Model file for the job. Use its own axes, mm. Coordinates: 2 decimals unless noted, no trailing zeros. Order: outer loops, then holes, each group sorted by start corner. A loop starts at its lowest first (then second) coordinate and runs counter-clockwise, first axis right, second up. Notation, with made-up numbers: (17.25, -2) -> (32.25, -2) arc R26 cw to (32.25, 24) -> close; hole circle Ø2 at (49, 4). An arc over 180 degrees is marked (long way). Use CSV: the item, a comma, the result in double quotes. Start each with the question number.
(1) Probe L1, parallel to Y at x = 1.25, z = 7; L2, parallel to Y at x = -2.25, z = 15.25; L3, parallel to Z at x = 3.75, y = 2.5. List the from-to ranges inside material, lowest first.
(2) Cut at C-C on z = 16. Write the cut outline in (x, y).
(3) Pin check, flat tips, straight feed: pin 1 Ø3 at (x, y) = (0.5, -7.5) entering from +Z; pin 2 Ø5 at (x, z) = (-3.5, 10.5) entering from +Y; pin 3 Ø3 at (y, z) = (0.61, 6.83) entering from -X; pin 4 Ø1 at (x, y) = (-1, 8.5) entering from -Z. Stop position of each tip, or through.
(4) Cut at B-B on z = 7.5. Write the cut outline in (x, y).
(5) Pull direction Z, two halves, no side cores. Call faces 1 (the flat face through (4.178, 3.3, 7)), 2 (the cylindrical face through (-1.74, 7.59, -0.32)): pulls with the +Z half, pulls with the -Z half, needs draft (parallel to the pull), parting line crosses it, or undercut.
(6) Cut at D-D on y = -5.5. Write the cut outline in (x, z), plus the area to 3 significant figures.
(7) Cut at A-A on y = -8. Write the cut outline in (x, z).
```python
from build123d import *

# Parameters (mm, degrees)
SKETCH1_R           = 2.5
BOSS_EXTRUDE1_DEPTH = 12
BOSS_EXTRUDE2_DEPTH = 12


with BuildPart() as part:
    # Sketch1 → Boss-Extrude1 (new body)
    with BuildSketch(Plane(origin=(4.177782817, 0, 0), x_dir=(0, 0, -1), z_dir=(1, 0, 0))):
        with BuildLine():
            ThreePointArc((5.17160003, 0.862151985), (3.024281035, 2.061571734), (0.581113459, 1.777813393))
            ThreePointArc((0.581113459, 1.777813393), (0.306322633, 2.922590425), (-0.144249976, 4.010252494))
            ThreePointArc((-0.144249976, 4.010252494), (1.999103081, 5.216745044), (3.031319401, 7.449258441))
            ThreePointArc((3.031319401, 7.449258441), (2.88255375, 7.658695012), (2.729338849, 7.864899014))
            ThreePointArc((2.729338849, 7.864899014), (0.28712005, 7.573087536), (-1.522655071, 5.907464347))
            ThreePointArc((-1.522655071, 5.907464347), (-2.417848576, 6.672090425), (-3.421681197, 7.287187589))
            ThreePointArc((-3.421681197, 7.287187589), (-2.396830677, 9.523091882), (-2.873988583, 11.935954691))
            ThreePointArc((-2.873988583, 11.935954691), (-3.11744625, 12.01795018), (-3.36260338, 12.094715262))
            ThreePointArc((-3.36260338, 12.094715262), (-5.16687741, 10.423134625), (-5.651987492, 8.011858032))
            ThreePointArc((-5.651987492, 8.011858032), (-6.825650183, 8.104271984), (-7.999312874, 8.011858032))
            ThreePointArc((-7.999312874, 8.011858032), (-8.484422956, 10.423134625), (-10.288696986, 12.094715262))
            ThreePointArc((-10.288696986, 12.094715262), (-10.533854115, 12.01795018), (-10.777311783, 11.935954691))
            ThreePointArc((-10.777311783, 11.935954691), (-11.254469689, 9.523091882), (-10.229619169, 7.287187589))
            ThreePointArc((-10.229619169, 7.287187589), (-11.23345179, 6.672090425), (-12.128645295, 5.907464347))
            ThreePointArc((-12.128645295, 5.907464347), (-13.938420416, 7.573087536), (-16.380639215, 7.864899014))
            ThreePointArc((-16.380639215, 7.864899014), (-16.533854115, 7.658695012), (-16.682619767, 7.449258441))
            ThreePointArc((-16.682619767, 7.449258441), (-15.650403447, 5.216745044), (-13.50705039, 4.010252494))
            ThreePointArc((-13.50705039, 4.010252494), (-13.957622999, 2.922590425), (-14.232413825, 1.777813393))
            ThreePointArc((-14.232413825, 1.777813393), (-16.675581401, 2.061571734), (-18.822900396, 0.862151985))
            ThreePointArc((-18.822900396, 0.862151985), (-18.825650183, 0.605271984), (-18.822900396, 0.348391984))
            ThreePointArc((-18.822900396, 0.348391984), (-16.675581401, -0.851027765), (-14.232413825, -0.567269425))
            ThreePointArc((-14.232413825, -0.567269425), (-13.957622999, -1.712046456), (-13.50705039, -2.799708525))
            ThreePointArc((-13.50705039, -2.799708525), (-15.650403447, -4.006201075), (-16.682619767, -6.238714473))
            ThreePointArc((-16.682619767, -6.238714473), (-16.533854115, -6.448151043), (-16.380639215, -6.654355045))
            ThreePointArc((-16.380639215, -6.654355045), (-13.938420416, -6.362543568), (-12.128645295, -4.696920378))
            ThreePointArc((-12.128645295, -4.696920378), (-11.23345179, -5.461546456), (-10.229619169, -6.07664362))
            ThreePointArc((-10.229619169, -6.07664362), (-11.254469689, -8.312547914), (-10.777311783, -10.725410722))
            ThreePointArc((-10.777311783, -10.725410722), (-10.533854115, -10.807406211), (-10.288696986, -10.884171294))
            ThreePointArc((-10.288696986, -10.884171294), (-8.484422956, -9.212590657), (-7.999312874, -6.801314064))
            ThreePointArc((-7.999312874, -6.801314064), (-6.825650183, -6.893728016), (-5.651987492, -6.801314064))
            ThreePointArc((-5.651987492, -6.801314064), (-5.16687741, -9.212590657), (-3.36260338, -10.884171294))
            ThreePointArc((-3.36260338, -10.884171294), (-3.11744625, -10.807406211), (-2.873988583, -10.725410722))
            ThreePointArc((-2.873988583, -10.725410722), (-2.396830677, -8.312547914), (-3.421681197, -6.07664362))
            ThreePointArc((-3.421681197, -6.07664362), (-2.417848576, -5.461546456), (-1.522655071, -4.696920378))
            ThreePointArc((-1.522655071, -4.696920378), (0.28712005, -6.362543568), (2.729338849, -6.654355045))
            ThreePointArc((2.729338849, -6.654355045), (2.88255375, -6.448151043), (3.031319401, -6.238714473))
            ThreePointArc((3.031319401, -6.238714473), (1.999103081, -4.006201075), (-0.144249976, -2.799708525))
            ThreePointArc((-0.144249976, -2.799708525), (0.306322633, -1.712046456), (0.581113459, -0.567269425))
            ThreePointArc((0.581113459, -0.567269425), (3.024281035, -0.851027765), (5.17160003, 0.348391984))
            ThreePointArc((5.17160003, 0.348391984), (5.174349817, 0.605271984), (5.17160003, 0.862151985))
        make_face()
        with Locations((-6.825650183, 0.605271984)):
            Circle(SKETCH1_R, mode=Mode.SUBTRACT)
    extrude(amount=-BOSS_EXTRUDE1_DEPTH)

    # Sketch2 → Boss-Extrude2 (add)
    with BuildSketch(Plane(origin=(4.177782817, 0, 0), x_dir=(0, 0, -1), z_dir=(1, 0, 0))):
        with BuildLine():
            ThreePointArc((-4.325650183, 0.605271984), (-4.453941938, 1.395841399), (-4.825650183, 2.105271984))
            Line((-4.825650183, 2.105271984), (-4.825650183, -0.894728016))
            ThreePointArc((-4.825650183, -0.894728016), (-4.453941938, -0.185297431), (-4.325650183, 0.605271984))
        make_face()
    extrude(amount=-BOSS_EXTRUDE2_DEPTH)


solid = part.part
```
Outcome:
1,L1,"-6.89 to -1.89, 3.1 to 8.1"
1,L2,"-6.71 to -3.63, -0.88 to 2.09, 4.84 to 7.92"
1,L3,"-0.43 to 5.19, 8.46 to 14.08"
2,outline,"(-7.82, -6.71) -> (4.18, -6.71) -> (4.18, -4.44) -> (-7.82, -4.44) -> close; (-7.82, -0.93) -> (4.18, -0.93) -> (4.18, 2.14) -> (-7.82, 2.14) -> close; (-7.82, 5.65) -> (4.18, 5.65) -> (4.18, 7.92) -> (-7.82, 7.92) -> close"
3,pin 1,"z = 16.68"
3,pin 2,"y = 12.09"
3,pin 3,"through"
3,pin 4,"z = 2.49"
4,outline,"(-7.82, -6.86) -> (4.18, -6.86) -> (4.18, -1.8) -> (-7.82, -1.8) -> close; (-7.82, 3.01) -> (4.18, 3.01) -> (4.18, 8.07) -> (-7.82, 8.07) -> close"
5,face 1,"needs draft"
5,face 2,"undercut"
6,outline,"(-7.82, -2.87) -> (4.18, -2.87) -> (4.18, 0.92) -> (-7.82, 0.92) -> close; (-7.82, 2.47) -> (4.18, 2.47) -> (4.18, 11.18) -> (-7.82, 11.18) -> close; (-7.82, 12.73) -> (4.18, 12.73) -> (4.18, 16.52) -> (-7.82, 16.52) -> close"
6,area,"196 mm2"
7,outline,"(-7.82, 2.45) -> (4.18, 2.45) -> (4.18, 5.61) -> (-7.82, 5.61) -> close; (-7.82, 8.04) -> (4.18, 8.04) -> (4.18, 11.21) -> (-7.82, 11.21) -> close"
